Autodesk Inventor part; units mm, degrees
ref_plane "YZ Plane" through (0, 0, 0) normal (1, 0, 0) x (0, 1, 0)
ref_plane "XZ Plane" through (0, 0, 0) normal (0, 1, 0) x (-1, 0, 0)
ref_plane "XY Plane" through (0, 0, 0) normal (0, 0, 1) x (1, 0, 0)
sketch "Sketch1" plane through (0, 0, 0) normal (0, 0, 1) x (1, 0, 0)
  line L0 (-18.0312, 10.7455) -> (26.9688, 10.7455)
  line L1 (26.9688, 10.7455) -> (26.9688, 0.7455)
  line L2 (26.9688, 0.7455) -> (-18.0312, 0.7455)
  line L3 (-18.0312, 0.7455) -> (-18.0312, 10.7455)
  circle A0 centre (-8.0312, 5.7455) radius 2.6
  circle A1 centre (16.9688, 5.7455) radius 2.6
  point P0 (0, 0)
  dimension "d0" = 5.2
  dimension "d1" = 5.2
  dimension "d2" = 10
  dimension "d3" = 5
  dimension "d4" = 5
  dimension "d5" = 10
  dimension "d6" = 45
  dimension "d7" = 10
  dimension "d8" = 25
extrude "Extrusion1" add sketch "Sketch1" along normal blind 15
sketch "Sketch2" plane through (0, 0, 15) normal (0, 0, 1) x (1, 0, 0)
  line L0 (-17.927, 2.0194) -> (26.9688, 2.0194)
  line L1 (26.9688, 2.0194) -> (26.9688, 0.7455)
  line L2 (26.9688, 0.7455) -> (-17.927, 0.7455)
  line L3 (-17.927, 0.7455) -> (-17.927, 2.0194)
  point P0 (0, 0)
extrude "Extrusion2" add sketch "Sketch2" along normal blind 5
sketch "Sketch3" plane through (0, 0, 15) normal (0, 0, 1) x (1, 0, 0)
  point P0 (0, 0)
sketch "Sketch4" plane through (0, 0, 15) normal (0, 0, 1) x (1, 0, 0)
  line L0 (5.4688, 5.0194) -> (3.4688, 5.0194)
  line L1 (3.4688, 5.0194) -> (3.4688, 7.0194)
  line L2 (3.4688, 7.0194) -> (5.4688, 7.0194)
  line L3 (5.4688, 7.0194) -> (5.4688, 5.0194)
  line L4 (26.9688, 2.0194) -> (-17.927, 2.0194)
  line L5 (26.9688, 2.0194) -> (26.9688, 10.7455)
  line L6 (-18.0312, 10.7455) -> (-18.0312, 0.7455)
  point P0 (0, 0)
  dimension "d13" = 2
  dimension "d14" = 3
  dimension "d15" = 21.5
  dimension "d16" = 2
  dimension "d17" = 21.5
extrude "Extrusion3" add sketch "Sketch4" along normal blind 5
sketch "Sketch5" plane through (3.4688, 5.0194, 15) normal (0, -1, 0) x (1, 0, 0)
  line L0 (2, 0) -> (2, 5)
  line L1 (0, 5) -> (2, 5)
  line L2 (2, 5) -> (2, 3)
  line L3 (2, 3) -> (0, 3)
  line L4 (0, 3) -> (0, 5)
  point P0 (-3.4688, -15)
  dimension "d20" = 2
extrude "Extrusion4" add sketch "Sketch5" along normal blind 4
fillet "Fillet1" radius 1 4 edges at (4.4688, 2.0194, 18) (4.4688, 5.0194, 18) (4.4688, 5.0194, 15) (4.5209, 2.0194, 15)
fillet "Fillet2" radius 1 2 edges at (4.4688, 7.0194, 20) (4.4688, 7.0194, 15)
properties part number "Slider"
The model under review builds one solid part; all positions refer to its coordinate system, in mm. A direction names the side the tool comes from. Give positions to 0.01 mm unless a question says otherwise; leave off trailing zeros. Order: outer loops, then holes, each group sorted by start corner. A loop starts at its lowest first (then second) coordinate and runs counter-clockwise, first axis right, second up. Notation, with made-up numbers: M 14.25,-6 L 49.25,-6 A11 ccw 49.25,-1 Z; hole C -29,-5.75 d10. An arc over 180 degrees is marked long. Answer in a Markdown table with one row per item. Add a question column.
1. To check wall thickness, follow line 1 along X through (y, z) = (7.25, 8.25); line 2 along Z through (x, y) = (25, 7); line 3 along X through (y, z) = (6.75, 18.5). State the ranges of each line that lie inside material, in increasing order.
2. Add section B-B on x = -6.5. State the section outline as (y, z) points.
3. For pin 1 Ø1.8 at (y, z) = (1.5, 18.5) entering from -X; pin 2 Ø4.5 at (x, z) = (4.5, 17.5) entering from +Y; pin 3 Ø3 at (x, y) = (16.97, 5.75) entering from +Z; pin 4 Ø1.5 at (x, y) = (-5.5, 8) entering from +Z, all flat-tipped, find the tip position at first contact; note any pin that passes through.
4. Add section A-A on y = 2.5. State the section outline as (x, z) points.
5. Add section D-D on x = -13.5. State the section outline as (y, z) points.
6. Add section C-C on y = 7.5. State the section outline as (x, z) points.
7. Machinability: for faces 1 (the flat face through (3.469, 5, 18)), 2 (the cylindrical face through (4.455, 2.305, 17.699)), 3 (the flat face through (-17.927, 1, 17)), 4 (the flat face through (5.469, 5, 18)), which of the approach directions +Z, -Z, +X, -X, +Y, -Y give a long, thin tool a straight path to every point of the face, cutting with its end or side? Answer none if there is none.
8. Mouldability with a two-part tool opening along Z and no side actions: class faces 5 (the flat face through (4.5, 5.019, 16.5)), 6 (the flat face through (4, 7.019, 17)), 7 (the cylindrical face through (4.483, 7.305, 15.301)) as released by +Z, released by -Z, zero draft, split by the parting line, or undercut.
The answers:
| question | item | result |
|---|---|---|
| 1 | line 1 | -18.03 to -10.15, -5.91 to 14.85, 19.09 to 26.97 |
| 1 | line 2 | 0 to 15 |
| 1 | line 3 | 3.47 to 5.47 |
| 2 | outline | M 0.75,0 L 3.64,0 L 3.64,15 L 3.02,15 A1 cw 2.02,16 L 2.02,20 L 0.75,20 Z; M 7.85,0 L 10.75,0 L 10.75,15 L 7.85,15 Z |
| 3 | pin 1 | x = -17.93 |
| 3 | pin 2 | y = 7.36 |
| 3 | pin 3 | through |
| 3 | pin 4 | z = 15 |
| 4 | outline | M -18.03,0 L 26.97,0 L 26.97,15.15 L -17.93,15.15 L -17.93,15 L -18.03,15 Z; M 3.47,17.85 L 5.47,17.85 L 5.47,20 L 3.47,20 Z |
| 5 | outline | M 0.75,0 L 10.75,0 L 10.75,15 L 3.02,15 A1 cw 2.02,16 L 2.02,20 L 0.75,20 Z |
| 6 | outline | M -18.03,0 L -9.95,0 L -9.95,15 L -18.03,15 Z; M -6.11,0 L 15.05,0 L 15.05,15 L 5.47,15 L 5.47,15.15 L 3.47,15.15 L 3.47,15 L -6.11,15 Z; M 18.89,0 L 26.97,0 L 26.97,15 L 18.89,15 Z |
| 7 | face 1 | +Z, -X, +Y |
| 7 | face 2 | +X, -X |
| 7 | face 3 | +Z, -X, +Y, -Y |
| 7 | face 4 | +Z, +X, +Y |
| 8 | face 5 | undercut |
| 8 | face 6 | zero draft |
| 8 | face 7 | released by +Z |
